Input: part model. Units: mm. Frame: model coordinates. A direction names the side the tool comes from. Round coordinates to 2 decimals unless told otherwise and drop trailing zeros. Write each loop counter-clockwise with the first axis right and the second up, starting at its lowest first coordinate (ties: lowest second). Pieces come first, ordered by that corner, then holes. Notation, with made-up numbers: (19.25, -13.5) -> (48.25, -13.5) arc R15 cw to (48.25, 11.5) -> close; hole circle Ø10 at (66, 5.5). An arc over 180 degrees is marked (long way). Write item = value, one per line.
```python
from build123d import *

# Parameters (mm, degrees)
F1_DEPTH = 40
F2_R     = 19.99999
F3_R     = 10
F4_DEPTH = 10


# Not quite as in the source:
# - a fillet or chamfer is up to 0.001 mm smaller than in the source, because OpenCascade refuses the exact size


with BuildPart() as f1:
    # F0 (on Front) → F1 (new body)
    with BuildSketch(Plane.XZ):
        Polygon((0, 18), (0, 0), (75, 0), (75, 10), (50, 10), (50, 18), (40, 18), (40, 10), (10, 10), (10, 18), align=None)
    extrude(amount=F1_DEPTH)

    # F2 (radius 20 in the source; OpenCascade refuses exactly that, so slightly less here)
    f2_edges = [f1.edges().sort_by_distance(p)[0] for p in [
        (75, -40, 5),
        (75, 0, 5),
    ]]
    fillet(f2_edges, radius=F2_R)

    # F3 (on face) → F4 (cut, through all)
    with BuildSketch(Plane.XY.offset(10)):
        with Locations((25, -20)):
            Circle(F3_R)
    extrude(amount=-F4_DEPTH, mode=Mode.SUBTRACT)


solid = f1.part
```
1) Draft query along X for faces 4 (the face through (35.2, -19.7, 10)), 5 (the face through (69.297, -6.014, 5.07)), 6 (the face through (27, -40, 7)). Return one class per face: +X half, -X half, draft (parallel to the pull), parting line (faces both ways), or undercut.
Solutions:
face_4 = undercut
face_5 = +X half
face_6 = draft
2) Cut plane D-D (z = 14.25). Return the cut outline in (x, y), and give its area (3 significant figures).
Solutions:
outline = (0, -40) -> (10, -40) -> (10, 0) -> (0, 0) -> close; (40, -40) -> (50, -40) -> (50, 0) -> (40, 0) -> close
area = 800 mm^2
3) Line query: L1, parallel to Y at x = 25, z = 5; L2, parallel to X at y = -29.5, z = 14.5; L3, parallel to Z at x = 67, y = -11. Output: solid intervals per line, ascending. Write a range as from..to.
Solutions:
L1 = -40..-30, -10..0
L2 = 0..10, 40..50
L3 = 0..10
4) Cut plane C-C (y = -17). Return the cut outline in (x, z).
Solutions:
outline = (0, 0) -> (15.46, 0) -> (15.46, 10) -> (10, 10) -> (10, 18) -> (0, 18) -> close; (34.54, 0) -> (74.77, 0) -> (74.77, 10) -> (50, 10) -> (50, 18) -> (40, 18) -> (40, 10) -> (34.54, 10) -> close
5) First-contact query: P1, Ø12, axis at x = 25, y = -20, coming from the +Z side; P2, Ø6.5, axis at y = -13, z = 12.5, coming from the +X side; P3, Ø4, axis at y = -17, z = 8, coming from the +X side (3 decimals); P4, Ø6, axis at x = 64.5, y = -28, coming from the +Z side. Flat tips, straight axial feed; report the tip coordinate or a pass-through.
Solutions:
P1 = through
P2 = 74.38
P3 = 74.975
P4 = 10
6) Access query for faces 1 (the face through (40, -20, 14)), 2 (the face through (60, -20, 10)), 3 (the face through (27, 0, 7)). Directions: +Z, -Z, +X, -X, +Y, -Y. A direction counts if a zero-diameter tool reaches every point of the face in a straight line with its end or side. Return the directions, or none.
Solutions:
face_1 = +Z, +Y, -Y
face_2 = +Z, +X, +Y, -Y
face_3 = +Z, -Z, +X, -X, +Y
7) Cut plane A-A (x = 25). Return the cut outline in (y, z).
Solutions:
outline = (-40, 0) -> (-30, 0) -> (-30, 10) -> (-40, 10) -> close; (-10, 0) -> (0, 0) -> (0, 10) -> (-10, 10) -> close
